```python
from build123d import *

# Parameters (mm, degrees)
SKETCH1_W                  = 50.8
SKETCH1_H                  = 145.6436
SKETCH1_R                  = 7.14375
BOSS_EXTRUDE1_DEPTH        = 22.225
CUT_EXTRUDE2_DEPTH         = 45.45
FILLET1_R                  = 3.175
CUT_EXTRUDE4_DEPTH         = 51.8
MIRROR3_COPY_1_DEPTH       = 45.45
MIRROR3_COPY_2_DEPTH       = 45.45
MIRROR3_COPY_3_DEPTH       = 51.8
F_10_24_TAPPED_HOLE1_D     = 3.7973
F_10_24_TAPPED_HOLE1_DEPTH = 14.986
F_10_24_TAPPED_HOLE1_TIP   = 1.140824014
FILLET2_R                  = 3.175


with BuildPart() as part:
    # Sketch1 → Boss-Extrude1 (new body, symmetric)
    with BuildSketch(Plane.XY):
        Rectangle(SKETCH1_W, SKETCH1_H)
        with Locations((0, 38.1)):
            Circle(SKETCH1_R, mode=Mode.SUBTRACT)
        with Locations((0, -38.1)):
            Circle(SKETCH1_R, mode=Mode.SUBTRACT)
    extrude(amount=BOSS_EXTRUDE1_DEPTH, both=True)

    # Sketch3 → Cut-Extrude2 (cut, through all)
    with BuildSketch(Plane.XY.offset(22.225)):
        with BuildLine():
            Line((19.05, 66.4718), (19.05, 0))
            Line((19.05, 0), (6.35, 0))
            ThreePointArc((6.35, 0), (5.499261314, 3.175), (3.175, 5.499261314))
            Line((3.175, 5.499261314), (3.175, 25.803277876))
            ThreePointArc((3.175, 25.803277876), (12.7, 38.1), (3.175, 50.396722124))
            Line((3.175, 50.396722124), (3.175, 66.4718))
            Line((3.175, 66.4718), (19.05, 66.4718))
        make_face()
    cut_extrude2 = extrude(amount=-CUT_EXTRUDE2_DEPTH, mode=Mode.SUBTRACT)

    # Mirror4: Cut-Extrude2 across plane
    add(cut_extrude2.mirror(Plane(origin=(0, 0, 0), x_dir=(0, 0, 1), z_dir=(1, 0, 0))), mode=Mode.SUBTRACT)

    # Mirror1: Cut-Extrude2 across plane
    add(cut_extrude2.mirror(Plane.ZX), mode=Mode.SUBTRACT)

    # Fillet1
    fillet1_edges = [part.edges().sort_by_distance(p)[0] for p in [
        (3.175, 50.396722124, 0),
        (19.05, 66.4718, 0),
        (-19.05, 66.4718, 0),
        (-3.175, 50.396722124, 0),
        (-25.4, 72.8218, 0),
        (19.05, -66.4718, 0),
        (25.4, 72.8218, 0),
        (25.4, -72.8218, 0),
        (-25.4, -72.8218, 0),
    ]]
    fillet(fillet1_edges, radius=FILLET1_R)

    # Sketch5 → Cut-Extrude4 (cut, through all)
    with BuildSketch(Plane(origin=(25.4, 0, 0), x_dir=(0, 0, -1), z_dir=(1, 0, 0))):
        Polygon((19.05, 72.8218), (22.225, 69.6468), (22.225, 72.8218), align=None)
    cut_extrude4 = extrude(amount=-CUT_EXTRUDE4_DEPTH, mode=Mode.SUBTRACT)

    # Mirror2: Cut-Extrude4 across plane
    add(cut_extrude4.mirror(Plane.XY), mode=Mode.SUBTRACT)

    # Mirror3: Cut-Extrude4 across plane
    add(cut_extrude4.mirror(Plane.ZX), mode=Mode.SUBTRACT)

    # Mirror3 copy 1 sketch → Mirror3 copy 1 (cut, through all)
    with BuildSketch(Plane(origin=(0, 0, 22.225), x_dir=(-1, 0, 0), z_dir=(0, 0, 1))):
        with BuildLine():
            Line((19.05, 66.4718), (19.05, 0))
            Line((19.05, 0), (6.35, 0))
            ThreePointArc((6.35, 0), (5.499261314, 3.175), (3.175, 5.499261314))
            Line((3.175, 5.499261314), (3.175, 25.803277876))
            ThreePointArc((3.175, 25.803277876), (12.7, 38.1), (3.175, 50.396722124))
            Line((3.175, 50.396722124), (3.175, 66.4718))
            Line((3.175, 66.4718), (19.05, 66.4718))
        make_face()
    extrude(amount=-MIRROR3_COPY_1_DEPTH, mode=Mode.SUBTRACT)

    # Mirror3 copy 2 sketch → Mirror3 copy 2 (cut, through all)
    with BuildSketch(Plane.XY.offset(22.225)):
        with BuildLine():
            Line((19.05, -66.4718), (19.05, 0))
            Line((19.05, 0), (6.35, 0))
            ThreePointArc((6.35, 0), (5.499261314, -3.175), (3.175, -5.499261314))
            Line((3.175, -5.499261314), (3.175, -25.803277876))
            ThreePointArc((3.175, -25.803277876), (12.7, -38.1), (3.175, -50.396722124))
            Line((3.175, -50.396722124), (3.175, -66.4718))
            Line((3.175, -66.4718), (19.05, -66.4718))
        make_face()
    extrude(amount=-MIRROR3_COPY_2_DEPTH, mode=Mode.SUBTRACT)

    # Mirror3 copy 3 sketch → Mirror3 copy 3 (cut, through all)
    with BuildSketch(Plane(origin=(25.4, 0, 0), x_dir=(0, 0, 1), z_dir=(1, 0, 0))):
        Polygon((19.05, 72.8218), (22.225, 69.6468), (22.225, 72.8218), align=None)
    extrude(amount=-MIRROR3_COPY_3_DEPTH, mode=Mode.SUBTRACT)

    # #10-24 Tapped Hole1
    with Locations(Plane.XY.offset(22.225)):
        with Locations((0, 0)):
            Hole(F_10_24_TAPPED_HOLE1_D / 2, depth=F_10_24_TAPPED_HOLE1_DEPTH)
            with Locations((0, 0, -(F_10_24_TAPPED_HOLE1_DEPTH + F_10_24_TAPPED_HOLE1_TIP / 2))):  # 118° drill point
                Cone(0, F_10_24_TAPPED_HOLE1_D / 2, F_10_24_TAPPED_HOLE1_TIP, mode=Mode.SUBTRACT)

    # Fillet2
    fillet2_edges = [part.edges().sort_by_distance(p)[0] for p in [
        (-3.175, -5.499261314, 0),
        (-3.175, -25.803277876, 0),
        (-3.175, -50.396722124, 0),
        (-3.175, -66.4718, 0),
        (-19.05, -66.4718, 0),
        (19.05, -66.4718, 0),
        (3.175, 5.499261314, 0),
        (3.175, 25.803277876, 0),
        (3.175, 66.4718, 0),
        (-3.175, 66.4718, 0),
        (-3.175, 25.803277876, 0),
        (-3.175, 5.499261314, 0),
        (3.175, -66.4718, 0),
        (3.175, -50.396722124, 0),
        (3.175, -25.803277876, 0),
        (3.175, -5.499261314, 0),
    ]]
    fillet(fillet2_edges, radius=FILLET2_R)


solid = part.part
```
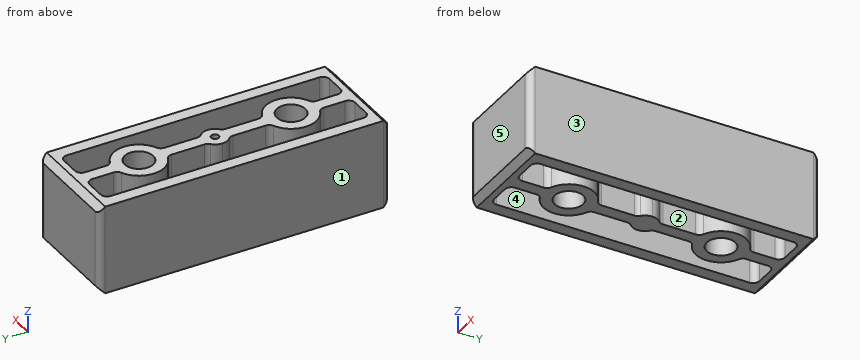
Could you check a few things on this model? Use its own coordinates, in mm. Face numbers are marked on the shaded views. A direction names the side the tool comes from. Coordinates: 2 decimals unless noted, no trailing zeros. Loops run counter-clockwise (first coordinate to the right, second up) from the corner with the lowest first, then second, coordinate; pieces in that order, holes last. Notation, with made-up numbers: M 7.25,-33.75 L 32.25,-33.75 A20 ccw 32.25,-9.75 Z; hole C 33.5,45 d11. An arc over 180 degrees is marked long. Put each result on its own line as item: value. Start each with the question number.
(1) Will this pin go through, and if not, where does the flat tip stop? P1, Ø2, axis at x = -13.5, y = -44.5, coming from the -Z side.
(2) I need wall thicknesses on line 1 (X direction, y = -55, z = 15) (3 decimals); line 2 (Y direction, x = 0, z = 11); line 3 (Y direction, x = 0, z = -3). Which ranges of each line are inside material? Lowest first, please. Write a range as from..to.
(3) For the marked faces 1 and 2, which set-ups out of +Z, -Z, +X, -X, +Y, -Y let a thin tool reach every point of the face, with its end or its side?
(4) Thinking about a two-plate mould opening in X: for the marked faces 3, 4 and 5, which applies, pulls with the +X half, pulls with the -X half, needs draft (parallel to the pull), parting line crosses it, or undercut?
(5) Suppose I cut it at A-A on y = -38.1. Please give me the cut outline in (x, z) (3 decimals), then the cut area to 3 significant figures.
(6) Suppose I cut it at B-B on y = -14. Please give me the cut outline in (x, z) (3 decimals), then the cut area to 3 significant figures.
(7) Suppose I cut it at C-C on z = 3.5. Count the separate pieces of the cut face and the enclosed holes in it, then the cut area to 3 significant figures.
Solutions:
1. P1: passes through
2. line 1: x = -25.4..-19.05, -3.175..3.175, 19.05..25.4
2. line 2: y = -72.82..-45.24, -30.96..-1.9, 1.9..30.96, 45.24..72.82
2. line 3: y = -72.82..-45.24, -30.96..30.96, 45.24..72.82
3. face 1: +Z, -Z, -X, +Y, -Y
3. face 2: +Z, -Z
4. face 3: pulls with the +X half
4. face 4: undercut
4. face 5: needs draft
5. outline: M -25.4,-22.225 L -19.05,-22.225 L -19.05,22.225 L -25.4,22.225 Z; M -12.7,-22.225 L -7.144,-22.225 L -7.144,22.225 L -12.7,22.225 Z; M 7.144,-22.225 L 12.7,-22.225 L 12.7,22.225 L 7.144,22.225 Z; M 19.05,-22.225 L 25.4,-22.225 L 25.4,22.225 L 19.05,22.225 Z
5. area: 1,060 mm2
6. outline: M -25.4,-22.225 L -19.05,-22.225 L -19.05,22.225 L -25.4,22.225 Z; M -3.175,-22.225 L 3.175,-22.225 L 3.175,22.225 L -3.175,22.225 Z; M 19.05,-22.225 L 25.4,-22.225 L 25.4,22.225 L 19.05,22.225 Z
6. area: 847 mm2
7. separate pieces: 1
7. enclosed holes: 4
7. area: 3,620 mm2
